Part model, mm, in its own coordinate system. Coordinates: 2 decimals unless noted, no trailing zeros. Order: outer loops, then holes, each group sorted by start corner. A loop starts at its lowest first (then second) coordinate and runs counter-clockwise, first axis right, second up.
1) Cut at A-A (z = 2.55). List the corners of the cut face in (x, y).
2) Wall check: L1, parallel to Y at x = 6.25, z = 2.7; L2, parallel to Z at x = -9, y = -7.75; L3, parallel to Y at x = -8, z = 0.6. Give the ranges that are in metal, low to high.
3) Cut at B-B (z = 0.55). List the corners of the cut face in (x, y) (1 decimal).
4) Pin check, flat tips, straight feed: pin 1 Ø1 at (y, z) = (10, 0.5) entering from +X; pin 2 Ø2 at (x, z) = (-2, 2.5) entering from +Y; pin 3 Ø16 at (x, y) = (0, 0) entering from +Z (3 decimals); pin 4 Ø1 at (x, z) = (-9, 0.5) entering from +Y. Stop position of each tip, or through.
```python
from build123d import *

# Parameters (mm, degrees)
F0_R     = 10
F1_DEPTH = 4
F2_R     = 1.99999
F3_R     = 1


# Not quite as in the source:
# - a fillet or chamfer is up to 0.001 mm smaller than in the source, because OpenCascade refuses the exact size


with BuildPart() as f1:
    # F0 (on Top) → F1 (new body)
    with BuildSketch(Plane.XY):
        Polygon((4.2186513593, -13.4238145334), (12.4751072696, -6.5090333023), (13.4238145334, 4.2186513593), (6.5090333023, 12.4751072696), (-4.2186513593, 13.4238145334), (-12.4751072696, 6.5090333023), (-13.4238145334, -4.2186513593), (-6.5090333023, -12.4751072696), align=None)
        Circle(F0_R, mode=Mode.SUBTRACT)
    extrude(amount=F1_DEPTH)

    # F2 (radius 2 in the source; OpenCascade refuses exactly that, so slightly less here)
    f2_edges = [f1.edges().sort_by_distance(p)[0] for p in [
        (-10, 0, 0),
        (-10, 0, 4),
    ]]
    fillet(f2_edges, radius=F2_R)

    # F3
    f3_edges = [f1.edges().sort_by_distance(p)[0] for p in [
        (1.145191, 12.949461, 4),
        (-8.346879, 9.966424, 4),
        (-12.949461, 1.145191, 4),
        (-9.966424, -8.346879, 4),
        (-1.145191, -12.949461, 4),
        (8.346879, -9.966424, 4),
        (12.949461, -1.145191, 4),
        (9.966424, 8.346879, 4),
        (9.966424, 8.346879, 0),
        (12.949461, -1.145191, 0),
        (8.346879, -9.966424, 0),
        (-1.145191, -12.949461, 0),
        (-9.966424, -8.346879, 0),
        (-12.949461, 1.145191, 0),
        (-8.346879, 9.966424, 0),
        (1.145191, 12.949461, 0),
    ]]
    fillet(f3_edges, radius=F3_R)


solid = f1.part
```
Geometry check:
1. outline: (-13.42, -4.22) - (-6.51, -12.48) - (4.22, -13.42) - (12.48, -6.51) - (13.42, 4.22) - (6.51, 12.48) - (-4.22, 13.42) - (-12.48, 6.51) - close; hole circle Ø20.15 at (0, 0)
2. L1: y = -11.72 to -7.97, 7.97 to 12.5
2. L2: z = 0 to 4
2. L3: y = -10.56 to -6.91, 6.91 to 10.15
3. outline: (-13.3, -4.2) - (-6.5, -12.4) - (4.2, -13.3) - (12.4, -6.5) - (13.3, 4.2) - (6.5, 12.4) - (-4.2, 13.3) - (-12.4, 6.5) - close; hole circle Ø21.2 at (0, 0)
4. pin 1: stops at x = 8.91
4. pin 2: stops at y = 13.32
4. pin 3: passes through
4. pin 4: stops at y = 9.74
